from build123d import *

# Parameters (mm, degrees)
F0_W     = 76.2
F0_H     = 50.8
F1_DEPTH = 12.7
F2_W     = 40
F2_H     = 0.39
F3_DEPTH = 25.4
F4_R     = 4.7625
F5_DEPTH = 25.4


with BuildPart() as f1:
    # F0 (on Top) → F1 (new body, symmetric)
    with BuildSketch(Plane.XY):
        Rectangle(F0_W, F0_H)
    extrude(amount=F1_DEPTH, both=True)

    # F2 (on face) → F3 (cut)
    with BuildSketch(Plane.XY.offset(12.7)):
        Polygon((-20, 0), (-20, 0.39), (20, 0.39), (20, 0), (38.1, 0), (38.1, 25.4), (-38.1, 25.4), (-38.1, 0), align=None)
        with Locations((0, 0.195)):
            Rectangle(F2_W, F2_H)
        with Locations((0, -0.195)):
            Rectangle(F2_W, F2_H)
    extrude(amount=-F3_DEPTH, mode=Mode.SUBTRACT)

    # F4 (on face) → F5 (cut)
    with BuildSketch(Plane.XZ.offset(25.4)):
        with Locations((-28.575, 0)):
            Circle(F4_R)
        with Locations((28.575, 0)):
            Circle(F4_R)
    extrude(amount=-F5_DEPTH, mode=Mode.SUBTRACT)


solid = f1.part
Could you check a few things on this model? Use its own coordinates, in mm. Coordinates: 2 decimals unless noted, no trailing zeros. Loops run counter-clockwise (first coordinate to the right, second up) from the corner with the lowest first, then second, coordinate; pieces in that order, holes last. Notation, with made-up numbers: (73.5, -16.75) -> (80.5, -16.75) arc R27 ccw to (80.5, 8.25) -> close; hole circle Ø5 at (75.25, 48). An arc over 180 degrees is marked (long way). Answer in a Markdown table with one row per item.
(1) Imagine slicing it at D-D (x = 2). List the corners of the cut face in (y, z) for me.
Results found:
| item | result |
|---|---|
| outline | (-25.4, -12.7) -> (-0.39, -12.7) -> (-0.39, 12.7) -> (-25.4, 12.7) -> close |
(2) If I drill on probe 1 along X at (y, z) = (-4.25, 2.25); probe 2 along Y at (x, z) = (-10.5, -8.75); probe 3 along Z at (x, y) = (-30.5, -5.75), over which ranges is the centre line in solid material (lowest first)?
Results found:
| item | result |
|---|---|
| probe 1 | x = -38.1 to -32.77, -24.38 to 24.38, 32.77 to 38.1 |
| probe 2 | y = -25.4 to -0.39 |
| probe 3 | z = -12.7 to -4.36, 4.36 to 12.7 |
(3) Imagine slicing it at C-C (y = -2). List the corners of the cut face in (x, z) for me (1 decimal).
Results found:
| item | result |
|---|---|
| outline | (-38.1, -12.7) -> (38.1, -12.7) -> (38.1, 12.7) -> (-38.1, 12.7) -> close; hole circle Ø9.5 at (-28.6, 0); hole circle Ø9.5 at (28.6, 0) |
(4) Imagine slicing it at B-B (x = -28). List the corners of the cut face in (y, z) for me, plus the area to 3 significant figures.
Results found:
| item | result |
|---|---|
| outline | (-25.4, -12.7) -> (0, -12.7) -> (0, -4.73) -> (-25.4, -4.73) -> close; (-25.4, 4.73) -> (0, 4.73) -> (0, 12.7) -> (-25.4, 12.7) -> close |
| area | 405 mm^2 |
(5) Will this pin go through, and if not, where does the flat tip stop? pin 1 Ø5.5 at (x, z) = (28.575, 0) entering from -Y.
Results found:
| item | result |
|---|---|
| pin 1 | passes through |
(6) Imagine slicing it at A-A (z = 0). List the corners of the cut face in (x, y) for me.
Results found:
| item | result |
|---|---|
| outline | (-38.1, -25.4) -> (-33.34, -25.4) -> (-33.34, 0) -> (-38.1, 0) -> close; (-23.81, -25.4) -> (23.81, -25.4) -> (23.81, 0) -> (20, 0) -> (20, -0.39) -> (-20, -0.39) -> (-20, 0) -> (-23.81, 0) -> close; (33.34, -25.4) -> (38.1, -25.4) -> (38.1, 0) -> (33.34, 0) -> close |
(7) Thinking about a two-plate mould opening in Z: for faces 1 (the face through (0, -0.39, 0)), 2 (the face through (23.817, -12.878, 0.209)), 3 (the face through (-1, -13, 12.7)), which applies, released by +Z, released by -Z, zero draft, split by the parting line, or undercut?
Results found:
| item | result |
|---|---|
| face 1 | zero draft |
| face 2 | undercut |
| face 3 | released by +Z |
